Autodesk Inventor part; units mm, degrees
ref_plane "YZ Plane" through (0, 0, 0) normal (1, 0, 0) x (0, 1, 0)
ref_plane "XZ Plane" through (0, 0, 0) normal (0, 1, 0) x (-1, 0, 0)
ref_plane "XY Plane" through (0, 0, 0) normal (0, 0, 1) x (1, 0, 0)
sketch "Sketch1" plane through (0, 0, 0) normal (0, 0, 1) x (1, 0, 0)
  line L0 (0, 0) -> (31.75, 0)
  line L1 (31.75, 0) -> (31.75, 25.4)
  line L2 (0, 25.4) -> (0, 0)
  line L3 (28.575, 25.4) -> (28.575, 3.175)
  line L4 (28.575, 3.175) -> (3.175, 3.175)
  line L5 (3.175, 3.175) -> (3.175, 25.4)
  line L6 (31.75, 25.4) -> (28.575, 25.4)
  line L7 (3.175, 25.4) -> (0, 25.4)
  dimension "d0" = 25.4
  dimension "d1" = 31.75
  dimension "d2" = 3.175
  dimension "d3" = 3.175
  dimension "d4" = 3.175
extrude "Extrusion1" add sketch "Sketch1" along normal blind 25.4
sketch "Sketch2" plane through (31.75, 0, 0) normal (1, 0, 0) x (0, 0, -1)
  line L0 (-25.4, 25.4) -> (-25.4, 0)
  line L1 (0, 0) -> (-25.4, 0)
  line L2 (0, 0) -> (0, 25.4)
  line L3 (0, 25.4) -> (-25.4, 25.4)
  circle A0 centre (-12.7, 12.7) radius 4.7625
  arc A1 (-5.4006, 15.818) -> (-19.9994, 15.818) centre (-12.7, 12.7) ccw
  line L4 (-19.9994, 15.818) -> (-25.4, 3.175)
  line L5 (-5.4006, 15.818) -> (0, 3.175)
  point P0 (0, 12.7)
  dimension "d9" = 9.525
  dimension "d13" = 3.175
  dimension "d14" = 12.7
  dimension "d15" = 7.9375
  dimension "d16" = 12.7
extrude "Extrusion2" cut sketch "Sketch2" against normal through all contours L3 L2 L5 A1 L4 L0 | A0
equation "\"d3\" = d2"
equation "\"d4\" = d3"
properties part number "manipulator pnumaitic pivot"
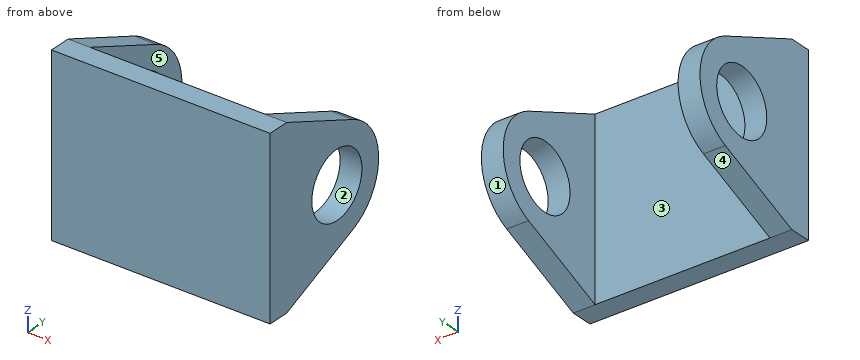
Source: CAD feature listing. Evaluate the final solid. Frame: model axes, mm. Face numbers are marked on the shaded views. A direction names the side the tool comes from. Round coordinates to 2 decimals unless told otherwise and drop trailing zeros. Loops run counter-clockwise (first coordinate to the right, second up) from the corner with the lowest first, then second, coordinate; pieces in that order, holes last. Notation, with made-up numbers: (35, 16.25) - (71, 16.25) arc R30 ccw to (71, 47.25) - close; hole circle Ø6 at (-23, 57). An arc over 180 degrees is marked (long way). Write item = value, one per line. Start each with the question number.
Item 1: Mould query, pull axis Z, two halves, no side actions, for the marked faces 1, 2 and 3. Classes: released by +Z, released by -Z, zero draft, split by the parting line, or undercut.
Item 2: Section query B-B on y = 4.25. Output: boundary loops of the cut face in (x, z) (3 decimals).
Item 3: First-contact query: pin 1 Ø5 at (y, z) = (9, 7) entering from -X; pin 2 Ø12.5 at (x, z) = (15, 16.5) entering from +Y (3 decimals); pin 3 Ø1 at (x, y) = (19, 5) entering from +Z. Flat tips, straight axial feed; report the tip coordinate or a pass-through.
Item 4: Section query D-D on x = 5.5. Output: boundary loops of the cut face in (y, z) (3 decimals), plus the area to 3 significant figures.
Item 5: Section query C-C on y = 12. Output: boundary loops of the cut face in (x, z) (3 decimals), plus the area to 3 significant figures.
Item 6: Section query A-A on z = 12.7. Count the separate pieces of the cut face and the enclosed holes in it, plus the area to 3 significant figures.
Item 7: Reachability of the marked faces 4 and 5 from +Z, -Z, +X, -X, +Y, -Y: full face, straight path, thin tool, end or side. Return the list, or none.
Item 8: Material intervals for line 1 (Y direction, x = 2.3, z = 12.7); line 2 (X direction, y = 5.25, z = 8) (3 decimals); line 3 (Y direction, x = 5.5, z = 19) (3 decimals), sorted ascending.
Results list:
q1.face_1 = split by the parting line
q1.face_2 = undercut
q1.face_3 = zero draft
q2.outline = (0, 0.459) - (3.175, 0.459) - (3.175, 24.941) - (0, 24.941) - close; (28.575, 0.459) - (31.75, 0.459) - (31.75, 24.941) - (28.575, 24.941) - close
q3.pin_1 = 0
q3.pin_2 = 3.175
q3.pin_3 = through
q4.outline = (0, 0) - (3.175, 0) - (3.175, 25.4) - (0, 25.4) - close
q4.area = 80.6 mm²
q5.outline = (0, 3.77) - (3.175, 3.77) - (3.175, 7.989) - (0, 7.989) - close; (0, 17.411) - (3.175, 17.411) - (3.175, 21.63) - (0, 21.63) - close; (28.575, 3.77) - (31.75, 3.77) - (31.75, 7.989) - (28.575, 7.989) - close; (28.575, 17.411) - (31.75, 17.411) - (31.75, 21.63) - (28.575, 21.63) - close
q5.area = 53.6 mm²
q6.separate_pieces = 3
q6.enclosed_holes = 0
q6.area = 151 mm²
q7.face_4 = -Z, +X, -X, +Y
q7.face_5 = +Z, -Z, +Y
q8.line_1 = 0 to 7.94, 17.46 to 20.64
q8.line_2 = 0 to 3.175, 28.575 to 31.75
q8.line_3 = 0 to 3.175
